```python
from build123d import *

# Parameters (mm, degrees)
SKETCH2_W                                      = 63.5
SKETCH2_H                                      = 12.7
BOSS_EXTRUDE1_DEPTH                            = 6.35
CBORE_FOR_4_SOCKET_HEAD_CAP_SCREW1_D           = 3.2639
CBORE_FOR_4_SOCKET_HEAD_CAP_SCREW1_CBORE_D     = 5.55752
CBORE_FOR_4_SOCKET_HEAD_CAP_SCREW1_CBORE_DEPTH = 2.8448
CUT_EXTRUDE1_DEPTH                             = 7.35


with BuildPart() as part:
    # Sketch2 → Boss-Extrude1 (new body)
    with BuildSketch(Plane(origin=(0, 0, 0), x_dir=(1, 0, 0), z_dir=(0, 1, 0))):
        with Locations((20.894224422, 2.49179868)):
            Rectangle(SKETCH2_W, SKETCH2_H)
    extrude(amount=BOSS_EXTRUDE1_DEPTH)

    # CBORE for #4 Socket Head Cap Screw1 (through all)
    with Locations(Plane.XY.offset(3.85820132)):
        with Locations((14.544224422, 3.175), (27.244224422, 3.175)):
            CounterBoreHole(CBORE_FOR_4_SOCKET_HEAD_CAP_SCREW1_D / 2, CBORE_FOR_4_SOCKET_HEAD_CAP_SCREW1_CBORE_D / 2, CBORE_FOR_4_SOCKET_HEAD_CAP_SCREW1_CBORE_DEPTH)

    # Sketch8 → Cut-Extrude1 (cut, through all)
    with BuildSketch(Plane(origin=(0, 6.35, 0), x_dir=(1, 0, 0), z_dir=(0, 1, 0))):
        with BuildLine():
            Line((-4.505775578, 5.66679868), (8.194224422, 5.66679868))
            ThreePointArc((8.194224422, 5.66679868), (11.369224422, 2.49179868), (8.194224422, -0.68320132))
            Line((8.194224422, -0.68320132), (-4.505775578, -0.68320132))
            ThreePointArc((-4.505775578, -0.68320132), (-7.680775578, 2.49179868), (-4.505775578, 5.66679868))
        make_face()
        with BuildLine():
            Line((33.594224422, 5.66679868), (46.294224422, 5.66679868))
            ThreePointArc((46.294224422, 5.66679868), (49.469224422, 2.49179868), (46.294224422, -0.68320132))
            Line((46.294224422, -0.68320132), (33.594224422, -0.68320132))
            ThreePointArc((33.594224422, -0.68320132), (30.419224422, 2.49179868), (33.594224422, 5.66679868))
        make_face()
    extrude(amount=-CUT_EXTRUDE1_DEPTH, mode=Mode.SUBTRACT)


solid = part.part
```
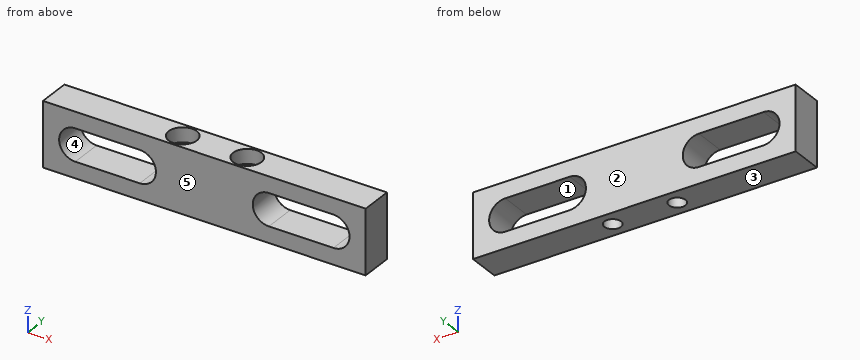
Work out the finished part from the listing and answer in its coordinate system (mm). Face numbers are marked on the shaded views. A direction names the side the tool comes from. Give positions to 0.01 mm unless a question says otherwise; leave off trailing zeros. Write each loop counter-clockwise with the first axis right and the second up, starting at its lowest first coordinate (ties: lowest second). Pieces come first, ordered by that corner, then holes. Notation, with made-up numbers: (62.5, 18.25) -> (72.5, 18.25) arc R33 cw to (72.5, 57.25) -> close; hole circle Ø1 at (39.5, -39). An arc over 180 degrees is marked (long way). Write item = value, one per line.
Q1. Section B-B on x = 27 is taken. Determine the outline of the cut face in (y, z), and give its area (3 significant figures).
Computed values:
outline = (0, -8.84) -> (1.56, -8.84) -> (1.56, 1.01) -> (0.41, 1.01) -> (0.41, 3.86) -> (0, 3.86) -> close; (4.79, -8.84) -> (6.35, -8.84) -> (6.35, 3.86) -> (5.94, 3.86) -> (5.94, 1.01) -> (4.79, 1.01) -> close
area = 33.1 mm^2
Q2. Section C-C on z = -5 is taken. Determine the outline of the cut face in (x, y) (3 decimals), and give its area (3 significant figures).
Computed values:
outline = (-10.856, 0) -> (-6.452, 0) -> (-6.452, 6.35) -> (-10.856, 6.35) -> close; (10.141, 0) -> (31.648, 0) -> (31.648, 6.35) -> (10.141, 6.35) -> close; (48.241, 0) -> (52.644, 0) -> (52.644, 6.35) -> (48.241, 6.35) -> close; hole circle Ø3.264 at (14.544, 3.175); hole circle Ø3.264 at (27.244, 3.175)
area = 176 mm^2
Q3. Section A-A on z = -1.25 is taken. Determine the outline of the cut face in (x, y) (3 decimals), and give its area (3 significant figures).
Computed values:
outline = (-10.856, 0) -> (-7.428, 0) -> (-7.428, 6.35) -> (-10.856, 6.35) -> close; (11.116, 0) -> (30.672, 0) -> (30.672, 6.35) -> (11.116, 6.35) -> close; (49.216, 0) -> (52.644, 0) -> (52.644, 6.35) -> (49.216, 6.35) -> close; hole circle Ø3.264 at (14.544, 3.175); hole circle Ø3.264 at (27.244, 3.175)
area = 151 mm^2
Q4. A flat-ended cylindrical pin translates along its axis: pin 1 Ø2 at (x, y) = (14.54, 3.18) entering from -Z. Find the tip coordinate at first contact, or state that the pin passes through.
Computed values:
pin_1 = through
Q5. For a pull along Z with two mould halves and no side action, classify the marked faces 1, 2 and 3 as pulls with the +Z half, pulls with the -Z half, needs draft (parallel to the pull), parting line crosses it, or undercut.
Computed values:
face_1 = undercut
face_2 = needs draft
face_3 = pulls with the -Z half
Q6. Consider line 1 along Y through (x, z) = (27, 2); line 2 along X through (y, z) = (5.5, 2.75); line 3 along X through (y, z) = (1.25, -1.25). Determine where each line is inside the solid, lowest interval first.
Computed values:
line_1 = 0 to 0.41, 5.94 to 6.35
line_2 = -10.86 to 13.02, 16.07 to 25.72, 28.77 to 52.64
line_3 = -10.86 to -7.43, 11.12 to 30.67, 49.22 to 52.64
Q7. Section D-D on x = 1.5 is taken. Determine the outline of the cut face in (y, z), and give its area (3 significant figures).
Computed values:
outline = (0, -8.84) -> (6.35, -8.84) -> (6.35, -5.67) -> (0, -5.67) -> close; (0, 0.68) -> (6.35, 0.68) -> (6.35, 3.86) -> (0, 3.86) -> close
area = 40.3 mm^2
Q8. A tool of negligible diameter and unlimited length cuts with its end or side. For the marked faces 4 and 5, from which of +Z, -Z, +X, -X, +Y, -Y can it reach the whole face along a straight path? Write none if from no direction.
Computed values:
face_4 = +Y, -Y
face_5 = +Z, -Z, +X, -X, -Y
